from build123d import *

# Parameters (mm, degrees)
SKETCH1_W          = 250
SKETCH1_H          = 250
BASE_DEPTH         = 14
SKETCH3_W          = 190
SKETCH3_H          = 230
CUT_EXTRUDE1_DEPTH = 10
FILLET1_R          = 5
FILLET2_R          = 5


with BuildPart() as part:
    # Sketch1 → Base (new body)
    with BuildSketch(Plane(origin=(0, 0, 0), x_dir=(1, 0, 0), z_dir=(0, 1, 0))):
        Rectangle(SKETCH1_W, SKETCH1_H)
    extrude(amount=BASE_DEPTH)

    # Sketch3 → Cut-Extrude1 (cut)
    with BuildSketch(Plane(origin=(0, 14, 0), x_dir=(1, 0, 0), z_dir=(0, 1, 0))):
        Rectangle(SKETCH3_W, SKETCH3_H)
    extrude(amount=-CUT_EXTRUDE1_DEPTH, mode=Mode.SUBTRACT)

    # Fillet1
    fillet1_edges = [part.edges().sort_by_distance(p)[0] for p in [
        (0, 0, 125),
        (-125, 0, 0),
        (0, 0, -125),
        (125, 0, 0),
    ]]
    fillet(fillet1_edges, radius=FILLET1_R)

    # Fillet2
    # the kernel refuses this fillet: 5 mm, written as the material it takes off along each edge
    with BuildSketch(Plane(origin=(120, 5, 120), x_dir=(1, 0, 0), z_dir=(0, 0, 1))) as fillet2_piece_1_section:
        Polygon((0, 0), (FILLET2_R, 0), (FILLET2_R, -FILLET2_R), (0, -FILLET2_R), align=None)
    fillet2_piece_1 = extrude(amount=FILLET2_R, mode=Mode.PRIVATE)
    fillet2_piece_1 = fillet2_piece_1 - Plane(origin=(120, 5, 120), x_dir=(-0.7071067811865475, 0.7071067811865475, 0), z_dir=(0, 0, 1)) * Sphere(FILLET2_R, mode=Mode.PRIVATE)
    add(fillet2_piece_1, mode=Mode.SUBTRACT)
    with BuildSketch(Plane(origin=(-120, 5, 120), x_dir=(-1, 0, 0), z_dir=(0, 0, 1))) as fillet2_piece_2_section:
        Polygon((0, 0), (FILLET2_R, 0), (FILLET2_R, FILLET2_R), (0, FILLET2_R), align=None)
    fillet2_piece_2 = extrude(amount=FILLET2_R, mode=Mode.PRIVATE)
    fillet2_piece_2 = fillet2_piece_2 - Plane(origin=(-120, 5, 120), x_dir=(0.7071067811865475, 0.7071067811865475, 0), z_dir=(0, 0, 1)) * Sphere(FILLET2_R, mode=Mode.PRIVATE)
    add(fillet2_piece_2, mode=Mode.SUBTRACT)
    with BuildSketch(Plane(origin=(120, 5, -120), x_dir=(0, 0, -1), z_dir=(1, 0, 0))) as fillet2_piece_3_section:
        Polygon((0, 0), (FILLET2_R, 0), (FILLET2_R, -FILLET2_R), (0, -FILLET2_R), align=None)
    fillet2_piece_3 = extrude(amount=FILLET2_R, mode=Mode.PRIVATE)
    fillet2_piece_3 = fillet2_piece_3 - Plane(origin=(120, 5, -120), x_dir=(0, 0.7071067811865475, 0.7071067811865475), z_dir=(1, 0, 0)) * Sphere(FILLET2_R, mode=Mode.PRIVATE)
    add(fillet2_piece_3, mode=Mode.SUBTRACT)
    with BuildSketch(Plane(origin=(-120, 5, -120), x_dir=(0, 0, -1), z_dir=(-1, 0, 0))) as fillet2_piece_4_section:
        Polygon((0, 0), (FILLET2_R, 0), (FILLET2_R, FILLET2_R), (0, FILLET2_R), align=None)
    fillet2_piece_4 = extrude(amount=FILLET2_R, mode=Mode.PRIVATE)
    fillet2_piece_4 = fillet2_piece_4 - Plane(origin=(-120, 5, -120), x_dir=(0, 0.7071067811865475, 0.7071067811865475), z_dir=(-1, 0, 0)) * Sphere(FILLET2_R, mode=Mode.PRIVATE)
    add(fillet2_piece_4, mode=Mode.SUBTRACT)
    with BuildSketch(Plane(origin=(125, 5, 125), x_dir=(-1, 0, 0), z_dir=(0, 1, 0)), Plane(origin=(125, 5, -125), x_dir=(0, 0, 1), z_dir=(0, 1, 0))) as fillet2_piece_5:
        with BuildLine():
            CenterArc((FILLET2_R, -FILLET2_R), FILLET2_R, 90, 90)
            Line((0, -FILLET2_R), (0, 0))
            Line((0, 0), (FILLET2_R, 0))
        make_face()
    extrude(amount=21.5, mode=Mode.SUBTRACT)
    with BuildSketch(Plane(origin=(-125, 5, 125), x_dir=(1, 0, 0), z_dir=(0, 1, 0)), Plane(origin=(-125, 5, -125), x_dir=(0, 0, 1), z_dir=(0, 1, 0))) as fillet2_piece_6:
        with BuildLine():
            CenterArc((FILLET2_R, FILLET2_R), FILLET2_R, 180, 90)
            Line((0, FILLET2_R), (0, 0))
            Line((0, 0), (FILLET2_R, 0))
        make_face()
    extrude(amount=21.5, mode=Mode.SUBTRACT)


solid = part.part
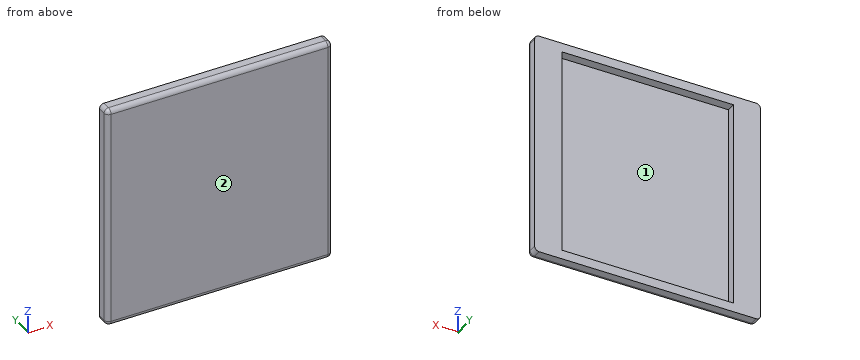
Can you work these out from the model? Positions are in its coordinate system, mm. Face numbers are marked on the shaded views. Coordinates: 2 decimals unless noted, no trailing zeros. Write each loop counter-clockwise with the first axis right and the second up, starting at its lowest first coordinate (ties: lowest second). Pieces come first, ordered by that corner, then holes. Notation, with made-up numbers: M -2,-22 L 23,-22 A25 ccw 23,11 Z; hole C -0.75,-20 d11. An arc over 180 degrees is marked long. Use one line per item in the form item = value.
Q1. If we section it at B-B (y = 7.25): Write out the boundary of the cut face in (x, z).
Model answer:
outline = M -125,-120 A5 ccw -120,-125 L 120,-125 A5 ccw 125,-120 L 125,120 A5 ccw 120,125 L -120,125 A5 ccw -125,120 Z; hole M -95,-115 L 95,-115 L 95,115 L -95,115 Z
Q2. We'd pull the mould along X, two halves only. Please class the marked faces 1 and 2: +X half, -X half, draft (parallel to the pull), parting line (faces both ways), or undercut.
Model answer:
face_1 = undercut
face_2 = draft
Q3. If we section it at A-A (x = 65.5): Write out the boundary of the cut face in (y, z).
Model answer:
outline = M 0,-120 A5 ccw 5,-125 L 14,-125 L 14,-115 L 4,-115 L 4,115 L 14,115 L 14,125 L 5,125 A5 ccw 0,120 Z
Q4. If we section it at C-C (z = -49): Write out the boundary of the cut face in (x, y).
Model answer:
outline = M -125,5 A5 ccw -120,0 L 120,0 A5 ccw 125,5 L 125,14 L 95,14 L 95,4 L -95,4 L -95,14 L -125,14 Z
Q5. For P1, Ø6, axis at x = -60, z = -13, coming from the +Y side; P2, Ø6, axis at x = -49, y = 4.5, coming from the +Z side, each with a flat end and sliding along its axis, tell me the tip position at first contact or that it passes through.
Model answer:
P1 = 4
P2 = 125
Q6. I need wall thicknesses on line 1 along X through (y, z) = (13.25, -93); line 2 along Z through (x, y) = (76, 6.5); line 3 along Z through (x, y) = (-4, 4.25). Which ranges of each line are inside material? Lowest first, please. Write a range as from..to.
Model answer:
line_1 = -125..-95, 95..125
line_2 = -125..-115, 115..125
line_3 = -124.94..-115, 115..124.94
